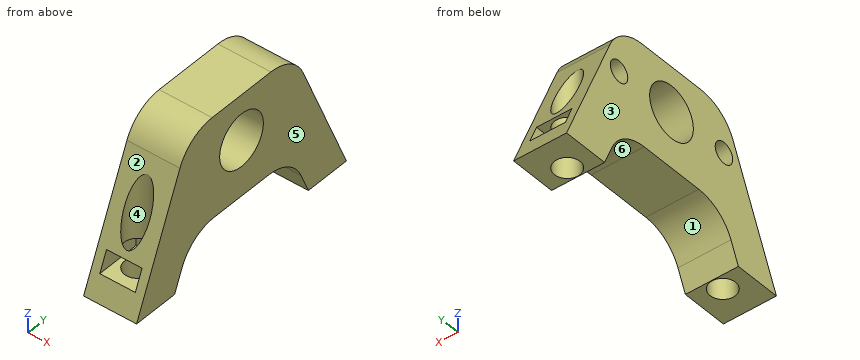
```python
from build123d import *

# Parameters (mm, degrees)
F1_DEPTH  = 25
F2_R      = 5
F3_DEPTH  = 15
F5_DEPTH  = 25
F7_W      = 16.75
F7_H      = 9
F8_DEPTH  = 25
F9_R      = 6
F10_DEPTH = 50
F11_R     = 20
F2_R_2    = 12.5
F12_DEPTH = 25


# Not quite as in the source:
# - a pattern or mirror of a feature is missing from the dataset's text; its kind, count and spacing are read off the source's solid


with BuildPart() as f1:
    # F0 (on Right) → F1 (new body)
    with BuildSketch(Plane.YZ):
        Polygon((-60, -35), (60, -35), (30, 35), (-30, 35), align=None)
    extrude(amount=F1_DEPTH)

    # F2 (on face) → F3 (cut)
    with BuildSketch(Plane(origin=(0, 0, 0), x_dir=(0, -1, 0), z_dir=(-1, 0, 0))):
        with Locations((-30, 13.5)):
            Circle(F2_R)
        with Locations((30, 13.5)):
            Circle(F2_R)
    extrude(amount=-F3_DEPTH, mode=Mode.SUBTRACT)

    # F4 (on face) → F5 (cut)
    with BuildSketch(Plane(origin=(0, 0, 0), x_dir=(0, -1, 0), z_dir=(-1, 0, 0))):
        Polygon((-28.8120768404, -13), (-38.240648269, -35), (38.240648269, -35), (28.8120768404, -13), align=None)
    extrude(amount=-F5_DEPTH, mode=Mode.SUBTRACT)

    # F7 (on offset) → F8 (cut)
    with BuildSketch(Plane.XZ.offset(60)):
        with Locations((12.5, -20.5)):
            Rectangle(F7_W, F7_H)
    f8 = extrude(amount=-F8_DEPTH, mode=Mode.SUBTRACT)

    # F8_copies: F8 across plane
    add(f8.mirror(Plane.ZX), mode=Mode.SUBTRACT)

    # F9 (on face) → F10 (cut, symmetric)
    with BuildSketch(Plane.XY.offset(-25)):
        with Locations((12.5, -44.487604307)):
            Circle(F9_R)
    f10 = extrude(amount=F10_DEPTH, both=True, mode=Mode.SUBTRACT)

    # F10_copies: F10 across plane
    add(f10.mirror(Plane.ZX), mode=Mode.SUBTRACT)

    # F11
    f11_edges = [f1.edges().sort_by_distance(p)[0] for p in [
        (12.5, -28.812077, -13),
        (12.5, 28.812077, -13),
        (12.5, 30, 35),
        (12.5, -30, 35),
    ]]
    fillet(f11_edges, radius=F11_R)

    # F2 (on face) → F12 (cut)
    with BuildSketch(Plane(origin=(0, 0, 0), x_dir=(0, -1, 0), z_dir=(-1, 0, 0))):
        with Locations((0, 13.5)):
            Circle(F2_R_2)
    extrude(amount=-F12_DEPTH, mode=Mode.SUBTRACT)


solid = f1.part
```
Model file for the job. Use its own axes, mm. Face numbers are marked on the shaded views. A direction names the side the tool comes from. Round coordinates to 2 decimals unless told otherwise and drop trailing zeros. Loops run counter-clockwise (first coordinate to the right, second up) from the corner with the lowest first, then second, coordinate; pieces in that order, holes last. Notation, with made-up numbers: M -1,-20 L 5,-20 A22 cw 5,4 Z; hole C 62.25,-24.5 d7. An arc over 180 degrees is marked long. Put each result on its own line as item: value. Start each with the question number.
Item 1: Cut at C-C (x = 13). Give the number of separate pieces and of enclosed holes in the cut face, then the cut area to 3 significant figures.
Item 2: 3-axis set-ups, long thin cutter, end or side, ignore diameter. For the marked faces 1 and 2: which of +Z, -Z, +X, -X, +Y, -Y reach the whole face in a straight line?
Item 3: Drill centre lines: line 1 along Z through (x, y) = (6.25, 0.5); line 2 along X through (y, z) = (-41.5, -20) (3 decimals); line 3 along Y through (x, z) = (8, -15.5). Where is each one in solid material? Low to high.
Item 4: Cut at A-A (y = 0). List the corners of the cut face in (x, z).
Item 5: Cut at D-D (y = 42.5). List the corners of the cut face in (x, z) (3 decimals).
Item 6: Drop flat-ended pins along their axis: P1, Ø5, axis at y = 28.5, z = 12, coming from the -X side; P2, Ø2, axis at x = 9.5, y = 23, coming from the -Z side; P3, Ø9.5, axis at x = 12.5, y = -44.49, coming from the -Z side; P4, Ø7, axis at x = 12, z = -22.5, coming from the -Y side. Give the stop position or say it passes through.
Item 7: Mould opens along X. For the marked faces 3, 4, 5 and 6 say: released by +X, released by -X, zero draft, split by the parting line, or undercut.
Item 8: Cut at B-B (z = 12). List the corners of the cut face in (x, y).
Answer block:
1. separate pieces: 5
1. enclosed holes: 3
1. area: 3,190 mm2
2. face 1: -Z, +X, -X
2. face 2: +Z, +X, -X, -Y
3. line 1: -13 to 1.01, 25.99 to 35
3. line 2: 0 to 4.125, 20.875 to 25
3. line 3: -51.64 to -48.46, -40.52 to -25.31, 25.31 to 40.52, 48.46 to 51.64
4. outline: M 0,-13 L 25,-13 L 25,1 L 0,1 Z; M 0,26 L 25,26 L 25,35 L 0,35 Z
5. outline: M 0,-35 L 6.839,-35 L 6.839,-25 L 4.125,-25 L 4.125,-16 L 6.839,-16 L 6.839,5.833 L 0,5.833 Z; M 18.161,-35 L 25,-35 L 25,5.833 L 18.161,5.833 L 18.161,-16 L 20.875,-16 L 20.875,-25 L 18.161,-25 Z
6. P1: x = 15
6. P2: z = -14.84
6. P3: through
6. P4: y = -56.14
7. face 3: released by -X
7. face 4: undercut
7. face 5: released by +X
7. face 6: zero draft
8. outline: M 0,-39.86 L 8.68,-39.86 A6 cw 16.32,-39.86 L 25,-39.86 L 25,-12.41 L 0,-12.41 L 0,-25.23 L 15,-25.23 L 15,-34.77 L 0,-34.77 Z; M 0,12.41 L 25,12.41 L 25,39.86 L 16.32,39.86 A6 cw 8.68,39.86 L 0,39.86 L 0,34.77 L 15,34.77 L 15,25.23 L 0,25.23 Z
